Source: three-view drawing plus pictorial views. Frame: mm from the lowest corner of the part. A direction names the side the tool comes from. Give positions to 0.01 mm unless a question says otherwise; leave off trailing zeros. Order: outer loops, then holes, each group sorted by start corner. A loop starts at its lowest first (then second) coordinate and runs counter-clockwise, first axis right, second up. Notation, with made-up numbers: (-18.5, 16) - (10.5, 16) arc R18 cw to (10.5, 41) - close; hole circle Ø7 at (37.25, -16). An arc over 180 degrees is marked (long way). Answer in a Markdown table with one row per item. Add a question column.
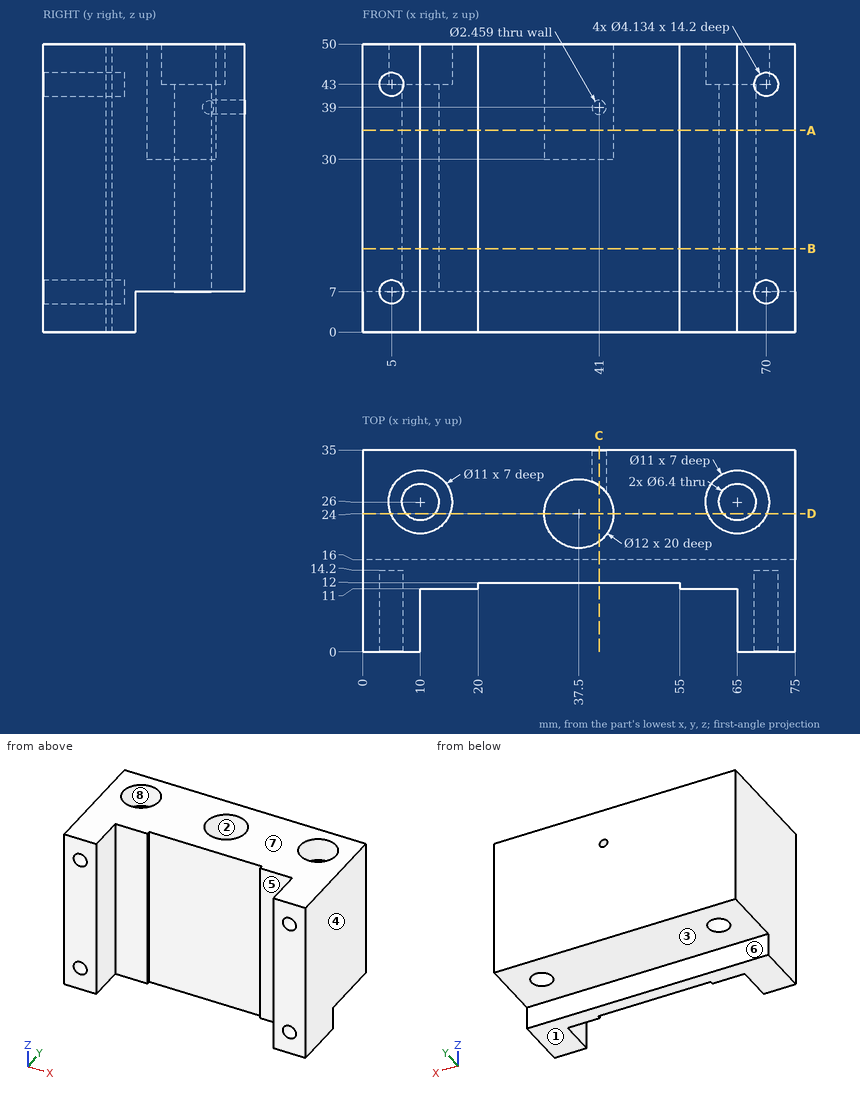
Q1. Section A-A, the plane z = 35. Return loops of the section in (x, y).
Q2. Pull-direction query (Y, two-part tool) for the marked faces 6, 7 and 8; classes: +Y half, -Y half, draft (parallel to the pull), parting line (faces both ways), or undercut.
Q3. Access query for the marked faces 1, 2, 3, 4 and 5. Directions: +Z, -Z, +X, -X, +Y, -Y. A direction counts if a zero-diameter tool reaches every point of the face in a straight line with its end or side. Return the directions, or none.
Q4. Section C-C, the plane x = 41. Return loops of the section in (y, z).
Q5. Section D-D, the plane y = 24. Return loops of the section in (x, z), then the cut area to 3 significant figures.
Q6. Section B-B, the plane z = 14.5. Return loops of the section in (x, y), then the cut area to 3 significant figures.
Q7. Contact query for flat-ended pins moving along their axis: P1, Ø19, axis at x = 37.5, y = 24, coming from the +Z side; P2, Ø10, axis at x = 33.5, z = 10.5, coming from the -Y side; P3, Ø3, axis at x = 54.5, y = 26.5, coming from the -Z side; P4, Ø5.5, axis at x = 9.5, y = 24, coming from the +Z side. Output: stop coordinate, or through.
Q8. Line query: probe 1 along Z at (x, y) = (70, 9); probe 2 along X at (y, z) = (8, 7); probe 3 along X at (y, z) = (26, 16). Output: solid intervals per line, ascending.
Computed:
| question | item | result |
|---|---|---|
| 1 | outline | (0, 0) - (10, 0) - (10, 11) - (20, 11) - (20, 12) - (55, 12) - (55, 11) - (65, 11) - (65, 0) - (75, 0) - (75, 35) - (0, 35) - close; hole circle Ø6.4 at (10, 26); hole circle Ø12 at (37.5, 24); hole circle Ø6.4 at (65, 26) |
| 2 | face 6 | +Y half |
| 2 | face 7 | draft |
| 2 | face 8 | undercut |
| 3 | face 1 | -Z, +X, -X, +Y, -Y |
| 3 | face 2 | +Z |
| 3 | face 3 | -Z, +X, -X, +Y |
| 3 | face 4 | +Z, -Z, +X, +Y, -Y |
| 3 | face 5 | +Z, -Z, -Y |
| 4 | outline | (12, 0) - (16, 0) - (16, 7) - (35, 7) - (35, 37.77) - (28.87, 37.77) - (28.87, 30) - (19.13, 30) - (19.13, 50) - (12, 50) - close; (28.87, 40.23) - (35, 40.23) - (35, 50) - (28.87, 50) - close |
| 5 | outline | (0, 7) - (7.5, 7) - (7.5, 43) - (4.88, 43) - (4.88, 50) - (0, 50) - close; (12.5, 7) - (62.5, 7) - (62.5, 43) - (59.88, 43) - (59.88, 50) - (43.5, 50) - (43.5, 30) - (31.5, 30) - (31.5, 50) - (15.12, 50) - (15.12, 43) - (12.5, 43) - close; (67.5, 7) - (75, 7) - (75, 50) - (70.12, 50) - (70.12, 43) - (67.5, 43) - close |
| 5 | area | 2,480 mm^2 |
| 6 | outline | (0, 0) - (10, 0) - (10, 11) - (20, 11) - (20, 12) - (55, 12) - (55, 11) - (65, 11) - (65, 0) - (75, 0) - (75, 35) - (0, 35) - close; hole circle Ø6.4 at (10, 26); hole circle Ø6.4 at (65, 26) |
| 6 | area | 1,920 mm^2 |
| 7 | P1 | stops at z = 50 |
| 7 | P2 | stops at y = 12 |
| 7 | P3 | stops at z = 7 |
| 7 | P4 | stops at z = 43 |
| 8 | probe 1 | z = 0 to 4.93, 9.07 to 40.93, 45.07 to 50 |
| 8 | probe 2 | x = 0 to 2.93, 7.07 to 10, 65 to 67.93, 72.07 to 75 |
| 8 | probe 3 | x = 0 to 6.8, 13.2 to 61.8, 68.2 to 75 |
